Work out the finished part from the listing and answer in its coordinate system (mm). A direction names the side the tool comes from. Round coordinates to 2 decimals unless told otherwise and drop trailing zeros. Write each loop counter-clockwise with the first axis right and the second up, starting at its lowest first coordinate (ties: lowest second). Pieces come first, ordered by that corner, then holes. Notation, with made-up numbers: (79, -23.5) -> (109, -23.5) arc R19 cw to (109, -3.5) -> close; hole circle Ø2 at (-3.75, 18). An arc over 180 degrees is marked (long way). Answer as a JSON object with one key per item and string values. Group by question number.
from build123d import *

# Parameters (mm, degrees)
F1_DEPTH = 5.8
F2_R     = 1.591325
F3_DEPTH = 25
F4_R     = 1.558187
F5_DEPTH = 24.1
F6_R     = 0.024142


with BuildPart() as f1:
    # F0 (on Top) → F1 (new body)
    with BuildSketch(Plane.XY):
        with BuildLine():
            ThreePointArc((-18.736619, 35.570893), (-18.046336, 36.984925), (-17.809047, 38.540454))
            ThreePointArc((-17.809047, 38.540454), (-25.090576, 43.331899), (-26.609889, 34.748759))
            ThreePointArc((-26.609889, 34.748759), (-22.484422, 33.351452), (-18.736619, 35.570893))
        make_face()
        with BuildLine():
            ThreePointArc((-18.736619, 35.570893), (-22.484422, 33.351452), (-26.609889, 34.748759))
            Line((-26.609889, 34.748759), (-29.543604, 34.748759))
            Line((-29.543604, 34.748759), (-29.543604, 25.887705))
            Line((-29.543604, 25.887705), (-29.543604, 16.994981))
            Line((-29.543604, 16.994981), (-25.393665, 16.994981))
            Line((-25.393665, 16.994981), (-20.255648, 16.994981))
            Line((-20.255648, 16.994981), (-15.710477, 16.994981))
            Line((-15.710477, 16.994981), (-15.710477, 28.654329))
            Line((-15.710477, 28.654329), (-15.710477, 32.804266))
            Line((-15.710477, 32.804266), (-15.710477, 35.570893))
            Line((-15.710477, 35.570893), (-18.736619, 35.570893))
        make_face()
        Polygon((-29.543604, 25.887705), (-29.543604, 34.748759), (-32.903075, 30.235259), (-50.886139, 30.235259), (-50.886139, 25.887705), align=None)
        Polygon((-6.980983, 32.804266), (-15.710477, 32.804266), (-15.710477, 28.654329), (-3.458281, 28.654329), (-3.458281, 40.511291), (-6.980983, 41.109147), align=None)
        Polygon((-25.393665, 16.994981), (-29.543604, 16.994981), (-29.543603, 2.766625), (-34.286387, 2.766625), (-34.286387, -1.185696), (-25.154444, -1.185696), align=None)
        with BuildLine():
            ThreePointArc((-52.614244, 26.742787), (-51.850182, 26.113168), (-50.886139, 25.887705))
            Line((-50.886139, 25.887705), (-50.886139, 30.235259))
            ThreePointArc((-50.886139, 30.235259), (-51.740629, 30.06027), (-52.457546, 29.563477))
            ThreePointArc((-52.457546, 29.563477), (-53.056569, 28.182057), (-52.614244, 26.742787))
        make_face()
        with BuildLine():
            Line((-68.671584, 28.061482), (-52.614244, 26.742787))
            ThreePointArc((-52.614244, 26.742787), (-53.056569, 28.182057), (-52.457546, 29.563477))
            Line((-52.457546, 29.563477), (-68.671584, 28.061482))
        make_face()
        Polygon((-15.710477, -1.185696), (-15.710477, 16.994981), (-20.255648, 16.994981), (-20.05803, 1.976161), (-23.229739, 1.934428), (-23.229739, -1.185696), align=None)
    extrude(amount=F1_DEPTH)

    # F2 (on face) → F3 (join)
    with BuildSketch(Plane.XZ.offset(1.185696)):
        with Locations((-30.139845, 3.054563)):
            Circle(F2_R)
    extrude(amount=F3_DEPTH)

    # F4 (on face) → F5 (join)
    with BuildSketch(Plane.XZ.offset(1.185696)):
        with Locations((-19.470108, 2.9)):
            Circle(F4_R)
    extrude(amount=F5_DEPTH)

    # F6
    f6_edges = [f1.edges().sort_by_distance(p)[0] for p in [
        (-15.710477, 13.734317, 5.8),
        (-9.584379, 28.654329, 5.8),
        (-3.458281, 34.58281, 5.8),
        (-3.458281, 34.58281, 0),
        (-23.568103, 43.729456, 5.8),
        (-28.076746, 34.748759, 5.8),
        (-31.223339, 32.492009, 5.8),
        (-41.894607, 30.235259, 5.8),
        (-51.740629, 30.06027, 5.8),
        (-60.564565, 28.812479, 5.8),
        (-60.642914, 27.402134, 5.8),
        (-51.850182, 26.113168, 5.8),
        (-40.214871, 25.887705, 5.8),
        (-29.543604, 21.441343, 5.8),
        (-29.543603, 9.880803, 5.8),
        (-31.914995, 2.766625, 5.8),
        (-34.286387, 0.790464, 5.8),
        (-29.720416, -1.185696, 5.8),
        (-25.274054, 7.904642, 5.8),
        (-22.824656, 16.994981, 5.8),
        (-20.156839, 9.485571, 5.8),
        (-21.643885, 1.955294, 5.8),
        (-23.229739, 0.374366, 5.8),
        (-19.470108, -1.185696, 5.8),
        (-5.219632, 40.810219, 5.8),
        (-6.980983, 36.956706, 5.8),
        (-11.34573, 32.804266, 5.8),
        (-15.710477, 34.18758, 5.8),
        (-17.223548, 35.570893, 5.8),
    ]]
    fillet(f6_edges, radius=F6_R)


solid = f1.part
1) Straight lines are drawn through the part: L1, parallel to Y at x = -8.5, z = 4.95; L2, parallel to Y at x = -17.5, z = 4; L3, parallel to X at y = 18.5, z = 4.3. For each, find the intervals that lie inside material, in ascending order.
2) Each of these flat-tipped pins is pushed along its axis until it touches: P1, Ø1.7, axis at y = 36, z = 4, coming from the -X side; P2, Ø0.9, axis at x = -18.5, z = 3.5, coming from the -Y side; P3, Ø3, axis at x = -12.5, z = 3.5, coming from the +Y side. Where does it stop, or does it pass through?
3) A cutting plane is placed at C-C on y = -6. Determine the outline of the cut face in (x, z), plus the area to 3 significant figures.
4) For a pull along Y with two mould halves and no side action, classify faces 1 (the face through (-28.62, -13.51, 3.53)), 2 (the face through (-28.8, -1.186, 1.6)), 3 (the face through (-23, 16.995, 3)) as released by +Y, released by -Y, zero draft, split by the parting line, or undercut.
5) A tool of negligible diameter and unlimited length cuts with its end or side. For faces 4 (the face through (-32, 2.767, 3)), 5 (the face through (-19, -25.286, 3)), 6 (the face through (-18.03, -13.07, 2.3)), 7 (the face through (-34.286, 1, 3)), 8 (the face through (-15.71, 34, 3)), from which of +Z, -Z, +X, -X, +Y, -Y can it reach the whole face along a straight path? Write none if from no direction.
Established:
{
 "1": {"L1": "y = 28.65 to 32.8", "L2": "y = -1.19 to 35.57", "L3": "x = -29.54 to -15.71"},
 "2": {"P1": "stops at x = -27.96", "P2": "stops at y = -25.29", "P3": "stops at y = 32.8"},
 "3": {"outline": "circle Ø3.18 at (-30.14, 3.05); circle Ø3.12 at (-19.47, 2.9)", "area": "15.6 mm²"},
 "4": {"face 1": "zero draft", "face 2": "released by -Y", "face 3": "undercut"},
 "5": {"face 4": "+Z, -Z, -X", "face 5": "+Z, -Z, +X, -Y", "face 6": "-Y", "face 7": "+Z, -Z, -X, -Y", "face 8": "+Z, -Z, +Y"}
}
